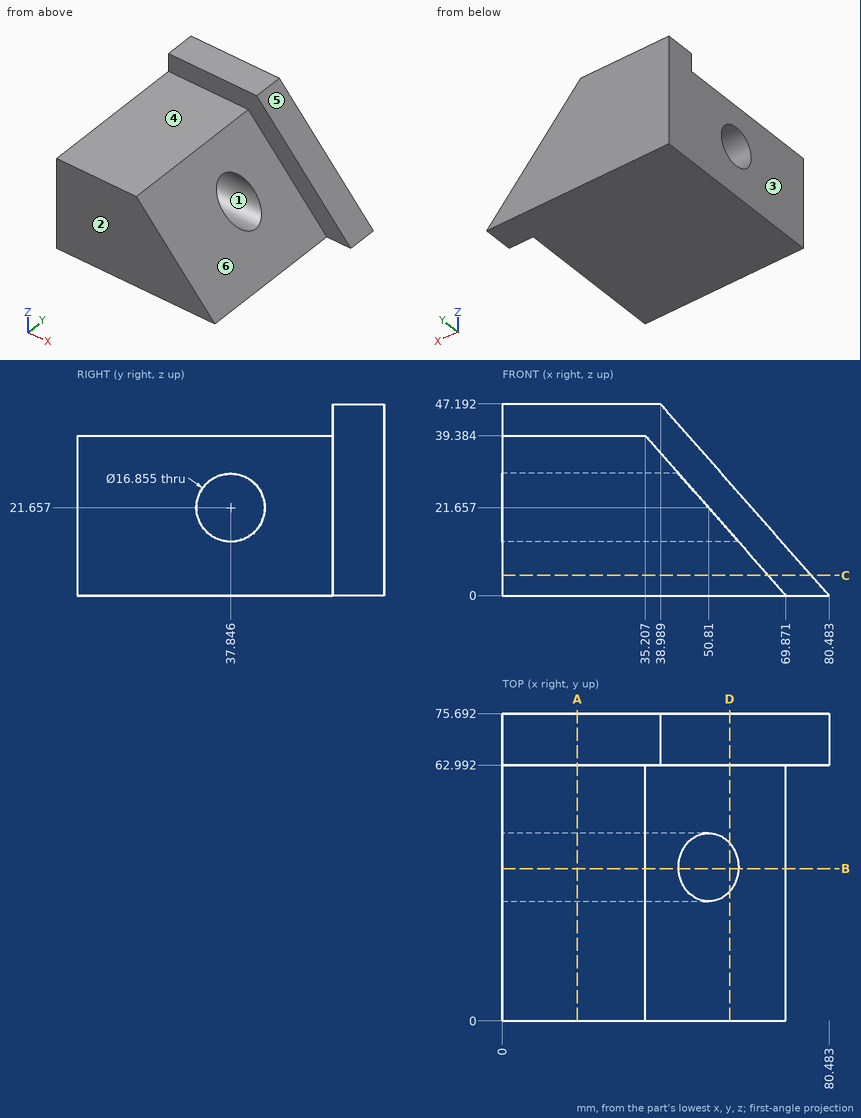
Input: dimensioned drawing with shaded views. Units: mm. Origin: part minimum x, y, z. A direction names the side the tool comes from. Coordinates: 2 decimals unless noted, no trailing zeros. Order: outer loops, then holes, each group sorted by start corner. A loop starts at its lowest first (then second) coordinate and runs counter-clockwise, first axis right, second up. Notation, with made-up numbers: M 48.5,80 L 73.5,80 A34 ccw 73.5,111 Z; hole C -1,85 d1. An arc over 180 degrees is marked long. Write each question's results on one line, items separated by ' | '. Start each with the question number.
Item 1: Cut plane B-B (y = 37.5). Return loops of the section in (x, z).
Item 2: Cut plane C-C (z = 5). Return loops of the section in (x, y), and give its area (3 significant figures).
Item 3: Draft query along Y for the marked faces 1, 2 and 3. Return one class per face: pulls with the +Y half, pulls with the -Y half, needs draft (parallel to the pull), parting line crosses it, or undercut.
Item 4: Cut plane D-D (x = 56). Return loops of the section in (y, z) (1 decimal).
Item 5: Cut plane A-A (x = 18.5). Return loops of the section in (y, z) (1 decimal), and give its area (3 significant figures).
Item 6: First-contact query: pin 1 Ø10 at (y, z) = (37.85, 21.66) entering from +X; pin 2 Ø2 at (x, y) = (68.5, 13) entering from +Z (1 decimal); pin 3 Ø1.5 at (y, z) = (12, 22.5) entering from +X; pin 4 Ø3 at (y, z) = (59.5, 32.5) entering from +X (1 decimal). Flat tips, straight axial feed; report the tip coordinate or a pass-through.
Item 7: Set-up query: the marked faces 4, 5 and 6. Return all of +Z, -Z, +X, -X, +Y, -Y with unobstructed straight access to the full face (end or side cutting, diameter ignored); none if empty.
Item 8: Line query: probe 1 along Z at (x, y) = (22, 37.5); probe 2 along Y at (x, z) = (63, 12); probe 3 along Z at (x, y) = (22.5, 28). Output: solid intervals per line, ascending.
Checked values:
1) outline: M 0,0 L 69.87,0 L 58.22,13.24 L 0,13.24 Z; M 0,30.08 L 43.4,30.08 L 35.21,39.38 L 0,39.38 Z
2) outline: M 0,0 L 65.47,0 L 65.47,62.99 L 76.09,62.99 L 76.09,75.69 L 0,75.69 Z | area: 5,090 mm2
3) face 1: undercut | face 2: pulls with the -Y half | face 3: needs draft
4) outline: M 0,0 L 75.7,0 L 75.7,27.8 L 63,27.8 L 63,15.8 L 43.9,15.8 A8.4 cw 31.8,15.8 L 0,15.8 Z
5) outline: M 0,0 L 75.7,0 L 75.7,47.2 L 63,47.2 L 63,39.4 L 0,39.4 Z; hole C 37.8,21.7 d16.9 | area: 2,860 mm2
6) pin 1: passes through | pin 2: stops at z = 2.7 | pin 3: stops at x = 50.73 | pin 4: stops at x = 42.6
7) face 4: +Z, +X, -X, -Y | face 5: +Z, +X, +Y, -Y | face 6: +Z, +X, -Y
8) probe 1: z = 0 to 13.24, 30.08 to 39.38 | probe 2: y = 62.99 to 75.69 | probe 3: z = 0 to 39.38
